```python
from build123d import *

# Parameters (mm, degrees)
BOSS_EXTRUDE1_DEPTH = 19.05


with BuildPart() as part:
    # Sketch1 → Boss-Extrude1 (new body)
    with BuildSketch(Plane(origin=(0, 0, 0), x_dir=(1, 0, 0), z_dir=(0, 1, 0))):
        with BuildLine():
            Line((-38.689871939, 17.78), (-29.890128061, 17.78))
            ThreePointArc((-29.890128061, 17.78), (-25.4, 17.78), (-25.4, 13.289871939))
            Line((-25.4, 13.289871939), (-25.4, 0))
            Line((-25.4, 0), (0, 0))
            Line((0, 0), (0, 25.4))
            Line((0, 25.4), (-14.2218161, 25.4))
            ThreePointArc((-14.2218161, 25.4), (-18.698135768, 25.048136767), (-19.05, 29.524456356))
            Line((-19.05, 29.524456356), (-19.05, 40.325543644))
            ThreePointArc((-19.05, 40.325543644), (-18.698136331, 44.801863892), (-14.2218161, 44.45))
            Line((-14.2218161, 44.45), (0, 44.45))
            Line((0, 44.45), (0, 76.2))
            Line((0, 76.2), (-14.2218161, 76.2))
            ThreePointArc((-14.2218161, 76.2), (-18.698136228, 75.848136228), (-19.05, 80.324456356))
            Line((-19.05, 80.324456356), (-19.05, 91.125543644))
            ThreePointArc((-19.05, 91.125543644), (-18.698136228, 95.601863772), (-14.2218161, 95.25))
            Line((-14.2218161, 95.25), (0, 95.25))
            Line((0, 95.25), (0, 120.65))
            Line((0, 120.65), (-25.4, 120.65))
            Line((-25.4, 120.65), (-25.4, 104.820128061))
            ThreePointArc((-25.4, 104.820128061), (-25.4, 100.33), (-29.890128061, 100.33))
            Line((-29.890128061, 100.33), (-41.229871939, 100.33))
            ThreePointArc((-41.229871939, 100.33), (-45.72, 100.33), (-45.72, 104.820128061))
            Line((-45.72, 104.820128061), (-45.72, 120.65))
            Line((-45.72, 120.65), (-77.47, 120.65))
            Line((-77.47, 120.65), (-77.47, 104.820128061))
            ThreePointArc((-77.47, 104.820128061), (-77.47, 100.33), (-81.960128061, 100.33))
            Line((-81.960128061, 100.33), (-93.299871939, 100.33))
            ThreePointArc((-93.299871939, 100.33), (-97.79, 100.33), (-97.79, 104.820128061))
            Line((-97.79, 104.820128061), (-97.79, 120.65))
            Line((-97.79, 120.65), (-116.84, 120.65))
            Line((-116.84, 120.65), (-116.84, 0))
            Line((-116.84, 0), (-92.71, 0))
            Line((-92.71, 0), (-92.71, 13.289871939))
            ThreePointArc((-92.71, 13.289871939), (-92.71, 17.78), (-88.219871939, 17.78))
            Line((-88.219871939, 17.78), (-79.420128061, 17.78))
            ThreePointArc((-79.420128061, 17.78), (-74.93, 17.78), (-74.93, 13.289871939))
            Line((-74.93, 13.289871939), (-74.93, 0))
            Line((-74.93, 0), (-43.18, 0))
            Line((-43.18, 0), (-43.18, 13.289871939))
            ThreePointArc((-43.18, 13.289871939), (-43.18, 17.78), (-38.689871939, 17.78))
        make_face()
    extrude(amount=BOSS_EXTRUDE1_DEPTH)


solid = part.part
```
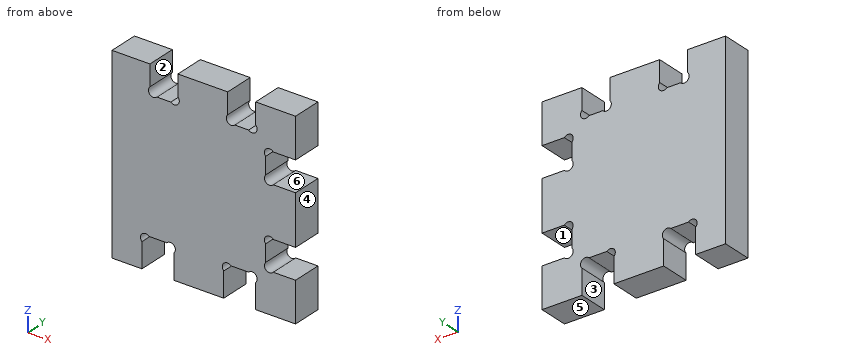
Model file for the job. Use its own axes, mm. Face numbers are marked on the shaded views. A direction names the side the tool comes from. Give positions to 0.01 mm unless a question says otherwise; leave off trailing zeros. Write each loop counter-clockwise with the first axis right and the second up, starting at its lowest first coordinate (ties: lowest second). Pieces come first, ordered by that corner, then holes. Notation, with made-up numbers: M 10,-34.75 L 67,-34.75 A4 cw 67,-30.75 Z; hole C 34.25,79 d4. An arc over 180 degrees is marked long. Use a Markdown table: item, result.
1) Pull direction Z, two halves, no side cores. Call the marked faces 4, 5 and 6: +Z half, -Z half, draft (parallel to the pull), parting line (faces both ways), or undercut.
Responses:
| item | result |
|---|---|
| face 4 | draft |
| face 5 | -Z half |
| face 6 | undercut |
2) Cut at A-A (x = -9). List the corners of the cut face in (y, z), and give its area (3 significant figures).
Responses:
| item | result |
|---|---|
| outline | M 0,-120.65 L 19.05,-120.65 L 19.05,-95.25 L 0,-95.25 Z; M 0,-76.2 L 19.05,-76.2 L 19.05,-44.45 L 0,-44.45 Z; M 0,-25.4 L 19.05,-25.4 L 19.05,0 L 0,0 Z |
| area | 1,570 mm2 |
3) Drill centre lines: line 1 (X direction, y = 14.5, z = -109); line 2 (Z direction, x = -10.5, y = 3.75); line 3 (X direction, y = 16, z = -16). Where is each one in solid material? Low to high. Write a range as from..to.
Responses:
| item | result |
|---|---|
| line 1 | x = -116.84..-97.79, -77.47..-45.72, -25.4..0 |
| line 2 | z = -120.65..-95.25, -76.2..-44.45, -25.4..0 |
| line 3 | x = -116.84..-93.61, -74.03..-44.08, -24.5..0 |
4) Tool access for the marked faces 1, 2 and 3: list every direction of +Z, -Z, +X, -X, +Y, -Y with a clear straight run to the whole face (end or side of a thin tool).
Responses:
| item | result |
|---|---|
| face 1 | +X, +Y, -Y |
| face 2 | +Z, +Y, -Y |
| face 3 | -Z, +Y, -Y |
5) Cut at B-B (z = -85.5). List the corners of the cut face in (x, y), and give its area (3 significant figures).
Responses:
| item | result |
|---|---|
| outline | M -116.84,0 L -19.05,0 L -19.05,19.05 L -116.84,19.05 Z |
| area | 1,860 mm2 |
6) Pin check, flat tips, straight feed: pin 1 (2 mm diameter, centred on x = -14.5, y = 10, fed in from +Z); pin 2 (2.5 mm diameter, centred on x = -85, y = 9.5, fed in from +Z); pin 3 (5.5 mm diameter, centred on x = -85, y = 11.5, fed in from -Z); pin 4 (6 mm diameter, centred on y = 7.5, z = -36, fed in from +X). Stop position of each tip, or through.
Responses:
| item | result |
|---|---|
| pin 1 | stops at z = 0 |
| pin 2 | stops at z = -17.78 |
| pin 3 | stops at z = -100.33 |
| pin 4 | stops at x = -19.05 |
